The model under review builds one solid part; all positions refer to its coordinate system, in mm. Round coordinates to 2 decimals unless told otherwise and drop trailing zeros. Write each loop counter-clockwise with the first axis right and the second up, starting at its lowest first coordinate (ties: lowest second). Pieces come first, ordered by that corner, then holes. Notation, with made-up numbers: (79, 66) -> (104, 66) arc R25 ccw to (104, 96) -> close; hole circle Ø5 at (59.5, 4). An arc over 180 degrees is marked (long way). Answer as a JSON object with one key per item and string values. Group by question number.
1) We need section A-A, the plane x = 0. Write out the cut boundary in (y, z).
2) Mouldability with a two-part tool opening along X and no side actions: class faces 1 (the flat face through (0, -10, 5)), 2 (the cylindrical face through (-0.26, -15.517, 2.465)), 3 (the cylindrical face through (10.382, -19.961, 2.465)) as pulls with the +X half, pulls with the -X half, needs draft (parallel to the pull), parting line crosses it, or undercut.
3) To check wall thickness, follow probe 1 along Y at (x, z) = (0, 1.1); probe 2 along X at (y, z) = (1.5, 1.3); probe 3 along Y at (x, z) = (-1, 4.4). State the ranges of each line that lie inside material, in increasing order. Write a range as [from, to].
4) We need section D-D, the plane y = 4.5. Write out the cut boundary in (x, z).
5) We need section C-C, the plane z = 2.8. Write out the cut boundary in (x, y).
from build123d import *

# Parameters (mm, degrees)
SKETCH_1_R               = 22.5
EXTRUDE_1_DEPTH          = 5
SKETCH_2_R               = 7.5
CUT_EXTRUDE_1_DEPTH      = 33.210246817
CUT_EXTRUDE_2_DEPTH      = 33.210246817
CUT_EXTRUDE_2_DEPTH_BACK = 33.210246817
SKETCH_3_R               = 2


with BuildPart() as part:
    # 草图1 → 凸台-拉伸1 (new body)
    with BuildSketch(Plane.XY):
        Circle(SKETCH_1_R)
    extrude(amount=EXTRUDE_1_DEPTH)

    # 草图2 → 切除-拉伸1 (cut, through all)
    with BuildSketch(Plane.XY.offset(5)):
        Circle(SKETCH_2_R)
    extrude(amount=-CUT_EXTRUDE_1_DEPTH, mode=Mode.SUBTRACT)

    # 草图3 → 切除-拉伸2 (cut, two sides: drawn at the far end of the back side and taken through both)
    with BuildSketch(Plane.XY.offset(5).offset(-CUT_EXTRUDE_2_DEPTH_BACK)):
        with Locations((-17.5, 0)):
            Circle(SKETCH_3_R)
        with Locations((0, -17.5)):
            Circle(SKETCH_3_R)
        with Locations((17.5, 0)):
            Circle(SKETCH_3_R)
        with Locations((0, 17.5)):
            Circle(SKETCH_3_R)
    extrude(amount=CUT_EXTRUDE_2_DEPTH + CUT_EXTRUDE_2_DEPTH_BACK, mode=Mode.SUBTRACT)


solid = part.part
Here are the results:
{
 "1": {"outline": "(-22.5, 0) -> (-19.5, 0) -> (-19.5, 5) -> (-22.5, 5) -> close; (-15.5, 0) -> (-7.5, 0) -> (-7.5, 5) -> (-15.5, 5) -> close; (7.5, 0) -> (15.5, 0) -> (15.5, 5) -> (7.5, 5) -> close; (19.5, 0) -> (22.5, 0) -> (22.5, 5) -> (19.5, 5) -> close"},
 "2": {"face 1": "needs draft", "face 2": "undercut", "face 3": "parting line crosses it"},
 "3": {"probe 1": "y = [-22.5, -19.5], [-15.5, -7.5], [7.5, 15.5], [19.5, 22.5]", "probe 2": "x = [-22.45, -18.82], [-16.18, -7.35], [7.35, 16.18], [18.82, 22.45]", "probe 3": "y = [-22.48, -19.23], [-15.77, -7.43], [7.43, 15.77], [19.23, 22.48]"},
 "4": {"outline": "(-22.05, 0) -> (-6, 0) -> (-6, 5) -> (-22.05, 5) -> close; (6, 0) -> (22.05, 0) -> (22.05, 5) -> (6, 5) -> close"},
 "5": {"outline": "circle Ø45 at (0, 0); hole circle Ø4 at (-17.5, 0); hole circle Ø15 at (0, 0); hole circle Ø4 at (0, -17.5); hole circle Ø4 at (0, 17.5); hole circle Ø4 at (17.5, 0)"}
}
